Design review of the part built by this model. Coordinates are the model's own, in mm. A direction names the side the tool comes from. Give positions to 0.01 mm unless a question says otherwise; leave off trailing zeros. Write each loop counter-clockwise with the first axis right and the second up, starting at its lowest first coordinate (ties: lowest second). Pieces come first, ordered by that corner, then holes. Notation, with made-up numbers: M 81.25,10.5 L 130.25,10.5 A19 ccw 130.25,29.5 Z; hole C 70,80.25 d8. An arc over 180 degrees is marked long. Write each question's results on one line, items separated by ' | '. Start each with the question number.
from build123d import *

# Parameters (mm, degrees)
F1_DEPTH = 12.7
F2_DEPTH = 6.35
F3_R     = 5.08
F4_R     = 5.08


with BuildPart() as f1:
    # F0 (on Top) → F1 (new body)
    with BuildSketch(Plane.XY):
        Polygon((-9.525, 44.45), (0, 63.5), (0, 76.2), (-19.05, 44.45), align=None)
        Polygon((0, 63.5), (9.525, 44.45), (19.05, 44.45), (0, 76.2), align=None)
        Polygon((9.525, 44.45), (12.7, 38.1), (12.7, -38.1), (9.525, -44.45), (19.05, -44.45), (19.05, 44.45), align=None)
        Polygon((-12.7, -38.1), (-12.7, 38.1), (-9.525, 44.45), (-19.05, 44.45), (-19.05, -44.45), (-9.525, -44.45), align=None)
        Polygon((0, -76.2), (0, -63.5), (-9.525, -44.45), (-19.05, -44.45), align=None)
        Polygon((19.05, -44.45), (9.525, -44.45), (0, -63.5), (0, -76.2), align=None)
    extrude(amount=F1_DEPTH)

    # F0 (on Top) → F2 (join)
    with BuildSketch(Plane.XY):
        Polygon((0, 38.1), (12.7, 38.1), (9.525, 44.45), (0, 44.45), align=None)
        Polygon((-12.7, 38.1), (0, 38.1), (0, 44.45), (-9.525, 44.45), align=None)
        Polygon((0, 44.45), (0, 63.5), (-9.525, 44.45), align=None)
        Polygon((0, 44.45), (9.525, 44.45), (0, 63.5), align=None)
        Polygon((12.7, -38.1), (12.7, 38.1), (0, 38.1), (-12.7, 38.1), (-12.7, -38.1), (0, -38.1), align=None)
        Polygon((0, -63.5), (9.525, -44.45), (0, -44.45), align=None)
        Polygon((-9.525, -44.45), (0, -63.5), (0, -44.45), align=None)
        Polygon((0, -44.45), (0, -38.1), (-12.7, -38.1), (-9.525, -44.45), align=None)
        Polygon((9.525, -44.45), (12.7, -38.1), (0, -38.1), (0, -44.45), align=None)
    extrude(amount=F2_DEPTH)

    # F3
    f3_edges = [f1.edges().sort_by_distance(p)[0] for p in [
        (19.05, -44.45, 6.35),
        (0, -76.2, 6.35),
        (-19.05, -44.45, 6.35),
        (-19.05, 44.45, 6.35),
        (0, 76.2, 6.35),
        (19.05, 44.45, 6.35),
    ]]
    fillet(f3_edges, radius=F3_R)

    # F4
    f4_edges = [f1.edges().sort_by_distance(p)[0] for p in [
        (-19.05, 0, 0),
    ]]
    fillet(f4_edges, radius=F4_R)


solid = f1.part
Q1. We need section B-B on y = -26.5. Write out the cut boundary in (x, z).
Q2. We need section A-A on z = 9. Write out the cut boundary in (x, y), and give its area (3 significant figures).
Q3. We need section C-C on z = 2.5. Write out the cut boundary in (x, y).
Q4. For faces 5 (the flat face through (12.7, 1, 9)), 6 (the cylindrical face through (10.1, -56.3, 1.4)), list the 3-axis set-ups (+Z, -Z, +X, -X, +Y, -Y) from which the entire face can be reached by the end or side of a thin tool; tool diameter is ignored.
Q5. For pin 1 Ø3 at (x, z) = (1, 1.5) entering from -Y; pin 2 Ø3 at (x, y) = (-8, -42) entering from +Z, all flat-tipped, find the tip position at first contact; note any pin that passes through.
Q6. Wall thickness on line 1 along X through (y, z) = (23, 11); line 2 along Z through (x, y) = (7.5, 43.5): over which ranges is each line inside the solid? List them lowest first. Write a range as from..to.
Q7. The part is to be moulded in two halves that separate along Y. For faces 1 (the cylindrical face through (-18.87, -44.38, 8.94)), 2 (the flat face through (-6.44, 50.62, 9.48)), 3 (the cylindrical face through (9.93, 56.68, 1.45)), 4 (the flat face through (6.44, -50.62, 9.48)), say which applies: pulls with the +Y half, pulls with the -Y half, needs draft (parallel to the pull), parting line crosses it, or undercut.
Answer sheet:
1) outline: M -19.05,5.08 A5.08 ccw -13.97,0 L 13.97,0 A5.08 ccw 19.05,5.08 L 19.05,12.7 L 12.7,12.7 L 12.7,6.35 L -12.7,6.35 L -12.7,12.7 L -19.05,12.7 Z
2) outline: M -19.05,-43.04 A5.08 ccw -18.33,-45.66 L -4.36,-68.94 A5.08 ccw 4.36,-68.94 L 18.33,-45.66 A5.08 ccw 19.05,-43.04 L 19.05,43.04 A5.08 ccw 18.33,45.66 L 4.36,68.94 A5.08 ccw -4.36,68.94 L -18.33,45.66 A5.08 ccw -19.05,43.04 Z; hole M -12.7,-38.1 L 0,-63.5 L 12.7,-38.1 L 12.7,38.1 L 0,63.5 L -12.7,38.1 Z | area: 1,980 mm^2
3) outline: M -18.35,-43.04 A4.38 ccw -17.72,-45.29 L -3.75,-68.58 A4.38 ccw 3.75,-68.58 L 17.72,-45.29 A4.38 ccw 18.35,-43.04 L 18.35,43.04 A4.38 ccw 17.72,45.29 L 3.75,68.58 A4.38 ccw -3.75,68.58 L -17.72,45.29 A4.38 ccw -18.35,43.04 Z
4) face 5: +Z | face 6: -Z, +X, -Y
5) pin 1: y = -70.9 | pin 2: z = 6.35
6) line 1: -19.05..-12.7, 12.7..19.05 | line 2: 0..6.35
7) face 1: pulls with the -Y half | face 2: undercut | face 3: pulls with the +Y half | face 4: undercut
